Could you check a few things on this model? Use its own coordinates, in mm. A direction names the side the tool comes from. Give positions to 0.01 mm unless a question says otherwise; leave off trailing zeros. Order: outer loops, then holes, each group sorted by start corner. A loop starts at its lowest first (then second) coordinate and runs counter-clockwise, first axis right, second up. Notation, with made-up numbers: (25.25, -35.5) - (40.25, -35.5) arc R29 cw to (40.25, -10.5) - close; hole circle Ø4 at (52.5, -10). An arc over 180 degrees is marked (long way). One line per question, with ' | ' between items. Start each with the question number.
1. Which directions (+Z, -Z, +X, -X, +Y, -Y) give clear straight access to the entire face, cutting with the end or side of a thin tool? Please do faces 1 (the flat face through (46, -25.4, 42)), 2 (the flat face through (41.275, -1, 4)), 3 (the flat face through (60, -2, 61.925)), 4 (the cylindrical face through (31.57, -16.79, 50.78)), 5 (the flat face through (-4, 7.938, 30)).
2. For P1, Ø5, axis at y = 19, z = 17.5, coming from the -X side (3 decimals); P2, Ø8, axis at x = 53.5, z = 43.5, coming from the +Y side; P3, Ø6, axis at x = 63, y = -0.5, coming from the -Z side; P4, Ø6, axis at x = 73.5, y = 25.5, coming from the +Z side (3 decimals), each with a flat end and sliding along its axis, tell me the tip position at first contact or that it passes through.
3. Imagine slicing it at A-A (y = 33.5). Please give me the cut outline in (x, z) (3 decimals), and give its area (3 significant figures).
4. If we mould it in two halves opening along X, with no side actions, what happens to faces 6 (the flat face through (46, 25.4, 42)), 7 (the flat face through (60, 2, 42.875)), 8 (the flat face through (22.225, 17, 18))? For each: released by +X, released by -X, zero draft, split by the parting line, or undercut.
5. I need wall thicknesses on probe 1 along Z at (x, y) = (-11.5, -54) (3 decimals); probe 2 along Y at (x, z) = (34, 24.5); probe 3 along Z at (x, y) = (104.5, 11.5) (3 decimals). Which ranges of each line are inside material? Lowest first, please. Write a range as from..to.
```python
from build123d import *

# Parameters (mm, degrees)
F1_DEPTH    = 89.68002
F0_W        = 25.4
F0_H        = 19.05
F2_DEPTH    = 25.4
F3_DEPTH    = 7.9375
F5_T1_DEPTH = 146.05


# Not quite as in the source:
# - a fillet or chamfer that OpenCascade refuses, or shapes differently, is made with other operations: its cross-section is extruded or revolved along the edge and cut away or added


with BuildPart() as f1:
    # F0 (on Front) → F1 (new body, symmetric)
    with BuildSketch(Plane.XZ):
        Polygon((22.225, 9.525), (-41.275, 9.525), (-41.275, -9.525), (41.275, -9.525), (41.275, 9.525), align=None)
    extrude(amount=F1_DEPTH, both=True)

    # F0 (on Front) → F2 (join, symmetric)
    with BuildSketch(Plane.XZ):
        with BuildLine():
            Line((22.225, 27.0002), (22.225, 9.525))
            Line((22.225, 9.525), (41.275, 9.525))
            Line((41.275, 9.525), (41.275, 27.0002))
            ThreePointArc((41.275, 27.0002), (45.9246798487, 38.2255201513), (57.15, 42.8752))
            Line((57.15, 42.8752), (60.325, 42.8752))
            Line((60.325, 42.8752), (60.325, 61.9252))
            Line((60.325, 61.9252), (57.15, 61.9252))
            add(Edge.make_bspline(
                [(53.8854342407, 61.7722898912), (54.9842067368, 61.8365871986), (56.0728453275, 61.8876096574), (57.15, 61.9252)],
                knots=[108.5245810491, 108.5245810491, 108.5245810491, 108.5245810491, 111.5045361635, 111.5045361635, 111.5045361635, 111.5045361635], degree=3))
            ThreePointArc((53.8854342407, 61.7722898912), (31.3258777096, 50.5133948686), (22.225, 27.0002))
        make_face()
        with Locations((73.025, 52.4002)):
            Rectangle(F0_W, F0_H)
    extrude(amount=F2_DEPTH, both=True)

    # F0 (on Front) → F3 (join, symmetric)
    with BuildSketch(Plane.XZ):
        with BuildLine():
            add(Edge.make_bspline(
                [(-41.275, 9.525), (-39.5856284224, 39.4828766469), (13.870125209, 59.4306981306), (53.8854342407, 61.7722898912)],
                knots=[0, 0, 0, 0, 108.5245810491, 108.5245810491, 108.5245810491, 108.5245810491], degree=3))
            Line((-41.275, 9.525), (22.225, 9.525))
            Line((22.225, 9.525), (22.225, 27.0002))
            ThreePointArc((22.225, 27.0002), (31.3258777096, 50.5133948686), (53.8854342407, 61.7722898912))
        make_face()
    extrude(amount=F3_DEPTH, both=True)

    # F0 (on Front) → F4 (revolve)
    with BuildSketch(Plane.XZ):
        Polygon((85.725, 66.675), (85.725, 61.9252), (85.725, 42.8752), (85.725, 38.1), (111.125, 38.1), (111.125, 66.675), align=None)
    revolve(axis=Axis((85.725, 0, 52.3875), (0, 0, 1)))

    # F5: fillet of radius 25.4 on 4 edges, made by hand

    # F5_s2 → F5_t1 (cut)
    with BuildSketch(Plane.XY.offset(-73.025)):
        with BuildLine():
            add(Edge.make_bspline(
                [(41.275, -64.28002), (41.275, -89.68002), (15.875, -89.68002)],
                knots=[0, 0, 0, 1, 1, 1], degree=2, weights=[1, 1, 1]))
            Line((15.875, -89.68002), (41.275, -89.68002))
            Line((41.275, -89.68002), (41.275, -64.28002))
        make_face()
        with BuildLine():
            add(Edge.make_bspline(
                [(-41.275, -64.28002), (-41.275, -89.68002), (-15.875, -89.68002)],
                knots=[0, 0, 0, 1, 1, 1], degree=2, weights=[1, 1, 1]))
            Line((-15.875, -89.68002), (-41.275, -89.68002))
            Line((-41.275, -89.68002), (-41.275, -64.28002))
        make_face()
        with BuildLine():
            add(Edge.make_bspline(
                [(41.275, 64.28002), (41.275, 89.68002), (15.875, 89.68002)],
                knots=[0, 0, 0, 1, 1, 1], degree=2, weights=[1, 1, 1]))
            Line((15.875, 89.68002), (41.275, 89.68002))
            Line((41.275, 89.68002), (41.275, 64.28002))
        make_face()
        with BuildLine():
            add(Edge.make_bspline(
                [(-41.275, 64.28002), (-41.275, 89.68002), (-15.875, 89.68002)],
                knots=[0, 0, 0, 1, 1, 1], degree=2, weights=[1, 1, 1]))
            Line((-15.875, 89.68002), (-41.275, 89.68002))
            Line((-41.275, 89.68002), (-41.275, 64.28002))
        make_face()
    extrude(amount=F5_T1_DEPTH, mode=Mode.SUBTRACT)


solid = f1.part
```
Results found:
1) face 1: +Z, +X, -X, -Y | face 2: -Z, +X, +Y, -Y | face 3: +Z, -X | face 4: +Z, -X, -Y | face 5: +Z, -X, +Y
2) P1: stops at x = 22.225 | P2: stops at y = 25.4 | P3: stops at z = 38.1 | P4: stops at z = 66.675
3) outline: (-41.275, -9.525) - (41.275, -9.525) - (41.275, 9.525) - (-41.275, 9.525) - close | area: 1,570 mm2
4) face 6: zero draft | face 7: undercut | face 8: released by -X
5) probe 1: z = -9.525..9.525 | probe 2: y = -25.4..25.4 | probe 3: z = 38.1..66.675
